```python
from build123d import *

# Parameters (mm, degrees)
SKETCH1_W           = 55
SKETCH1_H           = 36
SKETCH1_R           = 2
SKETCH1_R_2         = 3.5
SKETCH1_R_3         = 1.25
BOSS_EXTRUDE1_DEPTH = 1.5


with BuildPart() as part:
    # Sketch1 → Boss-Extrude1 (new, symmetric)
    with BuildSketch(Plane.XY):
        Rectangle(SKETCH1_W, SKETCH1_H)
        with Locations((-9, 13.5)):
            Circle(SKETCH1_R, mode=Mode.SUBTRACT)
        with Locations((-21, 9.5)):
            Circle(SKETCH1_R, mode=Mode.SUBTRACT)
        with Locations(Location((-9, -13.5, 0), (0, 0, 180))):
            Circle(SKETCH1_R, mode=Mode.SUBTRACT)
        with Locations(Location((-21, -9.5, 0), (0, 0, 180))):
            Circle(SKETCH1_R, mode=Mode.SUBTRACT)
        with Locations((9, -13.5)):
            Circle(SKETCH1_R, mode=Mode.SUBTRACT)
        with Locations((21, -9.5)):
            Circle(SKETCH1_R, mode=Mode.SUBTRACT)
        with Locations(Location((9, 13.5, 0), (0, 0, 180))):
            Circle(SKETCH1_R, mode=Mode.SUBTRACT)
        with Locations(Location((21, 9.5, 0), (0, 0, 180))):
            Circle(SKETCH1_R, mode=Mode.SUBTRACT)
        Circle(SKETCH1_R_2, mode=Mode.SUBTRACT)
        with Locations((0, 6.5)):
            Circle(SKETCH1_R_3, mode=Mode.SUBTRACT)
        with Locations((6.5, 0)):
            Circle(SKETCH1_R_3, mode=Mode.SUBTRACT)
        with Locations((0, -6.5)):
            Circle(SKETCH1_R_3, mode=Mode.SUBTRACT)
        with Locations((-6.5, 0)):
            Circle(SKETCH1_R_3, mode=Mode.SUBTRACT)
    extrude(amount=BOSS_EXTRUDE1_DEPTH, both=True)


solid = part.part
```
CAD build for the part. Positions are in the model's coordinates, mm. Coordinates: 2 decimals unless noted, no trailing zeros. Order: outer loops, then holes, each group sorted by start corner. A loop starts at its lowest first (then second) coordinate and runs counter-clockwise, first axis right, second up. Notation, with made-up numbers: (38, -21) -> (87, -21) arc R20 ccw to (87, -5) -> close; hole circle Ø3 at (35, -39.75). An arc over 180 degrees is marked (long way). Use one line per item in the form item = value. Start each with the question number.
1) Band-saw the part on B-B on y = -13.5. Give the cut face in (x, z), then the cut area to 3 significant figures.
2) Pull direction X, two halves, no side cores. Call faces 1 (the cylindrical face through (-22.474, 10.852, -0.021)), 2 (the flat face through (27.5, 0, 0)), 3 (the flat face through (0, 18, 0)), 4 (the flat face through (-27.5, 0, 0)): +X half, -X half, draft (parallel to the pull), parting line (faces both ways), or undercut.
3) Drop a flat-ended pin along its axis: pin 1 (3.5 mm diameter, centred on x = -21, y = -9.5, fed in from -Z). Give the stop position or say it passes through.
4) Drill centre lines: L1, parallel to Y at x = 0, z = -0.35; L2, parallel to Y at x = -9, z = -0.05; L3, parallel to Y at x = -10.5, z = 1.35. Where is each one in solid material? Low to high. Write a range as [from, to].
5) Band-saw the part on C-C on x = 9. Give the cut face in (y, z), then the cut area to 3 significant figures.
6) Band-saw the part on A-A on z = 0.25. State how many separate pieces and enclosed holes the cut face has, then the cut area to 3 significant figures.
7) Band-saw the part on D-D on y = 0. Give the cut face in (x, z), then the cut area to 3 significant figures.
Entries:
q1.outline = (-27.5, -1.5) -> (-11, -1.5) -> (-11, 1.5) -> (-27.5, 1.5) -> close; (-7, -1.5) -> (7, -1.5) -> (7, 1.5) -> (-7, 1.5) -> close; (11, -1.5) -> (27.5, -1.5) -> (27.5, 1.5) -> (11, 1.5) -> close
q1.area = 141 mm2
q2.face_1 = undercut
q2.face_2 = +X half
q2.face_3 = draft
q2.face_4 = -X half
q3.pin_1 = through
q4.L1 = [-18, -7.75], [-5.25, -3.5], [3.5, 5.25], [7.75, 18]
q4.L2 = [-18, -15.5], [-11.5, 11.5], [15.5, 18]
q4.L3 = [-18, -14.82], [-12.18, 12.18], [14.82, 18]
q5.outline = (-18, -1.5) -> (-15.5, -1.5) -> (-15.5, 1.5) -> (-18, 1.5) -> close; (-11.5, -1.5) -> (11.5, -1.5) -> (11.5, 1.5) -> (-11.5, 1.5) -> close; (15.5, -1.5) -> (18, -1.5) -> (18, 1.5) -> (15.5, 1.5) -> close
q5.area = 84.0 mm2
q6.separate_pieces = 1
q6.enclosed_holes = 13
q6.area = 1,820 mm2
q7.outline = (-27.5, -1.5) -> (-7.75, -1.5) -> (-7.75, 1.5) -> (-27.5, 1.5) -> close; (-5.25, -1.5) -> (-3.5, -1.5) -> (-3.5, 1.5) -> (-5.25, 1.5) -> close; (3.5, -1.5) -> (5.25, -1.5) -> (5.25, 1.5) -> (3.5, 1.5) -> close; (7.75, -1.5) -> (27.5, -1.5) -> (27.5, 1.5) -> (7.75, 1.5) -> close
q7.area = 129 mm2
